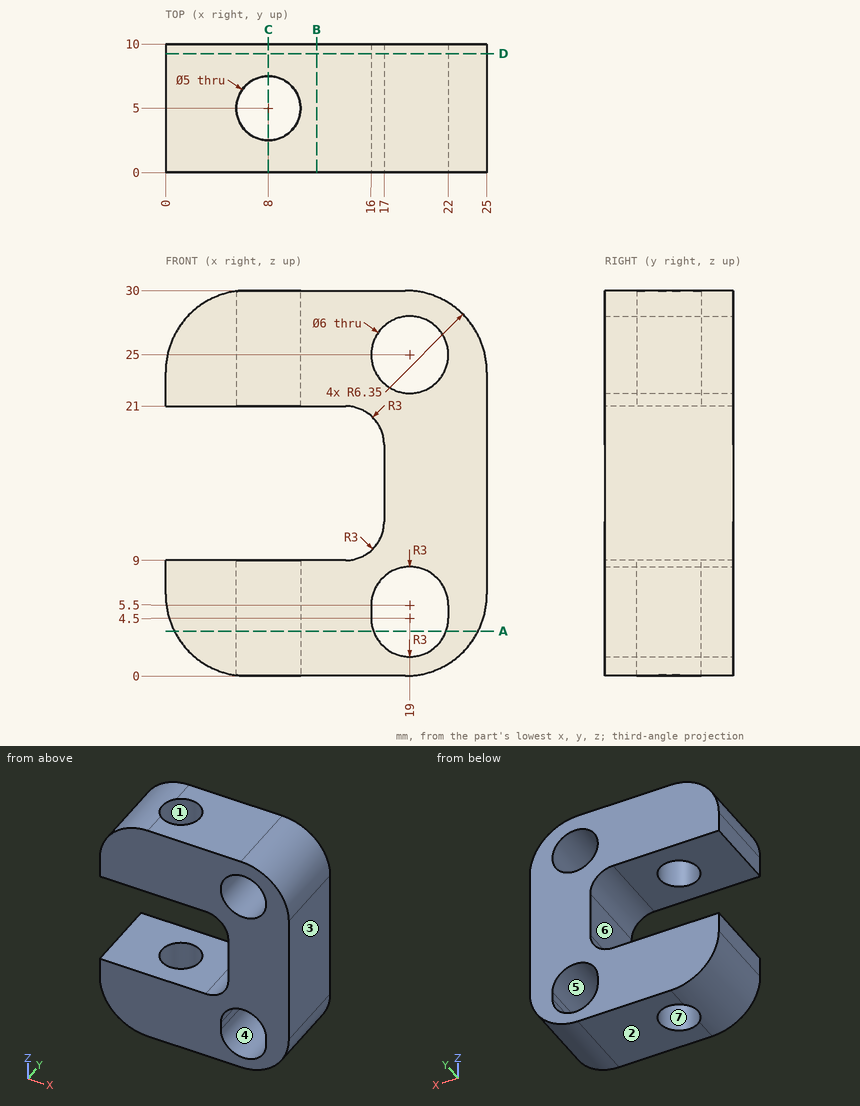
The drawing under review shows one solid part. Ordinate dimensions are in mm from its lowest x, y, z. A direction names the side the tool comes from. Round coordinates to 2 decimals unless told otherwise and drop trailing zeros. Loops run counter-clockwise (first coordinate to the right, second up) from the corner with the lowest first, then second, coordinate; pieces in that order, holes last. Notation, with made-up numbers: (78.25, -30) - (113.25, -30) arc R26 cw to (113.25, 5) - close; hole circle Ø6 at (77, 10). An arc over 180 degrees is marked (long way). Use one line per item in the form item = value.
Item 1: For line 1 (Z direction, x = 9.75, y = 8.5); line 2 (Z direction, x = 19, y = 5.5); line 3 (X direction, y = 7, z = 24), list the stretches that pass through material, from the lowest coordinate up.
Answers:
line_1 = 0 to 9, 21 to 30
line_2 = 0.01 to 1.5, 8.5 to 22, 28 to 29.99
line_3 = 0.01 to 6.5, 9.5 to 16.17, 21.83 to 24.99
Item 2: Consider section B-B on x = 11.75. Write out the cut boundary in (y, z).
Answers:
outline = (0, 0) - (10, 0) - (10, 9) - (0, 9) - close; (0, 21) - (10, 21) - (10, 30) - (0, 30) - close
Item 3: Mouldability with a two-part tool opening along X and no side actions: class the marked faces 1, 2, 3 and 4 as +X half, -X half, draft (parallel to the pull), parting line (faces both ways), or undercut.
Answers:
face_1 = undercut
face_2 = draft
face_3 = +X half
face_4 = undercut
Item 4: Consider section D-D on y = 9.25. Write out the cut boundary in (x, z).
Answers:
outline = (0, 6.35) arc R6.35 ccw to (6.35, 0) - (18.65, 0) arc R6.35 ccw to (25, 6.35) - (25, 23.65) arc R6.35 ccw to (18.65, 30) - (6.35, 30) arc R6.35 ccw to (0, 23.65) - (0, 21) - (14, 21) arc R3 cw to (17, 18) - (17, 12) arc R3 cw to (14, 9) - (0, 9) - close; hole (16, 4.5) arc R3 ccw to (22, 4.5) - (22, 5.5) arc R3 ccw to (16, 5.5) - close; hole circle Ø6 at (19, 25)
Item 5: Clearance check with flat-ended pins moving along their axes: P1, Ø1.1, axis at y = 4.5, z = 5, coming from the -X side; P2, Ø3, axis at y = 5, z = 15.5, coming from the -X side; P3, Ø1.5, axis at x = 4.5, y = 9, coming from the -Z side. State where each tip first meets the part, or that it passes through.
Answers:
P1 = 0.05
P2 = 17
P3 = 0.1
Item 6: Tool access review of the marked faces 5, 6 and 7: name each direction out of +Z, -Z, +X, -X, +Y, -Y from which nothing blocks a thin tool from reaching the whole face with its end or side.
Answers:
face_5 = +Y, -Y
face_6 = -X, +Y, -Y
face_7 = +Z, -Z
Item 7: Consider section C-C on x = 8. Write out the cut boundary in (y, z), then the cut area to 3 significant figures.
Answers:
outline = (0, 0) - (2.5, 0) - (2.5, 9) - (0, 9) - close; (0, 21) - (2.5, 21) - (2.5, 30) - (0, 30) - close; (7.5, 0) - (10, 0) - (10, 9) - (7.5, 9) - close; (7.5, 21) - (10, 21) - (10, 30) - (7.5, 30) - close
area = 90.0 mm^2
Item 8: Consider section A-A on z = 3.5. Write out the cut boundary in (x, y).
Answers:
outline = (0.68, 0) - (16.17, 0) - (16.17, 10) - (0.68, 10) - close; (21.83, 0) - (24.32, 0) - (24.32, 10) - (21.83, 10) - close; hole circle Ø5 at (8, 5)
